from build123d import *

# Parameters (mm, degrees)
SKETCH1_W           = 100
SKETCH1_H           = 40
BOSS_EXTRUDE2_DEPTH = 5
SKETCH4_R           = 3
CUT_EXTRUDE6_DEPTH  = 10
FLEX3_START         = 1.366197724
FLEX3_OUTLINE_W     = 5
FLEX3_OUTLINE_H     = 40
FLEX3_DEPTH         = 48.633802276
FLEX3_START_2       = -3.633802276
FLEX3_2_OUTLINE_W   = 46.366197724
FLEX3_2_OUTLINE_H   = 40
FLEX3_2_OUTLINE_R   = 3
FLEX3_2_DEPTH       = 3.907802276
FLEX3_START_3       = -5
FLEX3_3_OUTLINE_W   = 46.366197724
FLEX3_3_OUTLINE_H   = 40
FLEX3_3_OUTLINE_R   = 3
FLEX3_3_DEPTH       = 6.366197724
FLEX3_START_4       = -40
FLEX3_4_DEPTH       = 40
BOSS_EXTRUDE3_DEPTH = 1.5
CUT_EXTRUDE7_START  = -43
CUT_EXTRUDE7_DEPTH  = 43
BOSS_EXTRUDE4_DEPTH = 1.5
CUT_EXTRUDE8_DEPTH  = 40


with BuildPart() as part:
    # Sketch1 → Boss-Extrude2 (new body)
    with BuildSketch(Plane(origin=(0, 0, 0), x_dir=(1, 0, 0), z_dir=(0, 1, 0))):
        with Locations((0, 20)):
            Rectangle(SKETCH1_W, SKETCH1_H)
    extrude(amount=BOSS_EXTRUDE2_DEPTH)

    # Sketch4 → Cut-Extrude6 (cut)
    with BuildSketch(Plane(origin=(0, 5, 0), x_dir=(1, 0, 0), z_dir=(0, 1, 0))):
        with Locations(Location((-35, 30, 0), (0, 0, 270))):
            Circle(SKETCH4_R)
        with Locations(Location((-35, 10, 0), (0, 0, 270))):
            Circle(SKETCH4_R)
        with Locations(Location((35, 10, 0), (0, 0, 270))):
            Circle(SKETCH4_R)
        with Locations(Location((35, 30, 0), (0, 0, 270))):
            Circle(SKETCH4_R)
    extrude(amount=-CUT_EXTRUDE6_DEPTH, mode=Mode.SUBTRACT)

    # Flex3: read off the stored shape, not the designer's step
    # Flex3 outline → Flex3 (cut)
    with BuildSketch(Plane.YZ.offset(FLEX3_START)):
        with Locations((2.5, -20)):
            Rectangle(FLEX3_OUTLINE_W, FLEX3_OUTLINE_H)
    extrude(amount=FLEX3_DEPTH, mode=Mode.SUBTRACT)

    # Flex3 2 outline → Flex3 2 (add)
    with BuildSketch(Plane.YZ.offset(FLEX3_START_2)):
        with Locations((28.183098862, -20)):
            Rectangle(FLEX3_2_OUTLINE_W, FLEX3_2_OUTLINE_H)
        with Locations((36.366197724, -30)):
            Circle(FLEX3_2_OUTLINE_R, mode=Mode.SUBTRACT)
        with Locations((36.366197724, -10)):
            Circle(FLEX3_2_OUTLINE_R, mode=Mode.SUBTRACT)
    extrude(amount=FLEX3_2_DEPTH)

    # Flex3 3 outline → Flex3 3 (add)
    with BuildSketch(Plane.YZ.offset(FLEX3_START_3)):
        with Locations((28.183098862, -20)):
            Rectangle(FLEX3_3_OUTLINE_W, FLEX3_3_OUTLINE_H)
        with Locations((36.366197724, -30)):
            Circle(FLEX3_3_OUTLINE_R, mode=Mode.SUBTRACT)
        with Locations((36.366197724, -10)):
            Circle(FLEX3_3_OUTLINE_R, mode=Mode.SUBTRACT)
    extrude(amount=FLEX3_3_DEPTH)

    # Flex3 4 outline → Flex3 4 (cut)
    with BuildSketch(Plane.XY.offset(FLEX3_START_4)):
        with BuildLine():
            Line((1.366197724, 0), (1.366197724, 6.366197724))
            ThreePointArc((1.366197724, 6.366197724), (-0.498418419, 1.864616143), (-5, 0))
            Line((-5, 0), (1.366197724, 0))
        make_face()
        with BuildLine():
            ThreePointArc((-5, 5), (-4.033952325, 5.400150049), (-3.633802276, 6.366197724))
            Line((-3.633802276, 6.366197724), (-3.633802276, 51.366197724))
            Line((-3.633802276, 51.366197724), (-5, 51.366197724))
            Line((-5, 51.366197724), (-5, 5))
        make_face()
    extrude(amount=FLEX3_4_DEPTH, mode=Mode.SUBTRACT)

    # Sketch6 → Boss-Extrude3 (add, symmetric)
    with BuildSketch(Plane.XY.offset(-10)):
        Polygon((0, 0), (0, 15), (-15, 0), align=None)
    extrude(amount=BOSS_EXTRUDE3_DEPTH, both=True)

    # Sketch7 → Cut-Extrude7 (cut)
    with BuildSketch(Plane.XY.offset(CUT_EXTRUDE7_START)):
        with BuildLine():
            Line((-5, 0), (0, 0))
            Line((0, 0), (0, 2.425579313))
            ThreePointArc((0, 2.425579313), (-2.221356671, 0.638404544), (-5, 0))
        make_face()
    extrude(amount=CUT_EXTRUDE7_DEPTH, mode=Mode.SUBTRACT)

    # Sketch9 → Boss-Extrude4 (add, symmetric)
    with BuildSketch(Plane.XY.offset(-30)):
        Polygon((0, 0), (0, 15), (-15, 0), align=None)
    extrude(amount=BOSS_EXTRUDE4_DEPTH, both=True)

    # Sketch10 → Cut-Extrude8 (cut)
    with BuildSketch(Plane(origin=(0, 0, -40), x_dir=(-1, 0, 0), z_dir=(0, 0, -1))):
        with BuildLine():
            Line((0, 2.425579313), (0, 0))
            Line((0, 0), (5, 0))
            ThreePointArc((5, 0), (2.221356671, 0.638404544), (0, 2.425579313))
        make_face()
    extrude(amount=-CUT_EXTRUDE8_DEPTH, mode=Mode.SUBTRACT)


solid = part.part
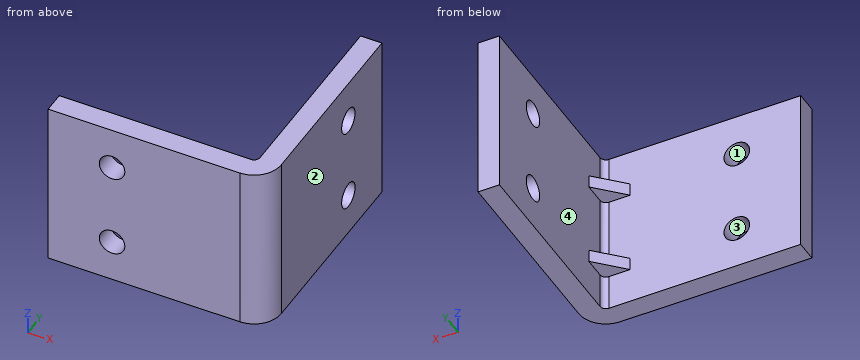
Input: part model. Units: mm. Frame: model coordinates. Face numbers are marked on the shaded views. Coordinates: 2 decimals unless noted, no trailing zeros. Loops run counter-clockwise (first coordinate to the right, second up) from the corner with the lowest first, then second, coordinate; pieces in that order, holes last. Notation, with made-up numbers: (86.5, -10) -> (110.5, -10) arc R20 cw to (110.5, -4) -> close; hole circle Ø4 at (62.25, -26). An arc over 180 degrees is marked (long way). One line per item, written item: value.
(1) Cut plane B-B (x = -35). Output: boundary loops of the cut face in (y, z).
Answer below:
outline: (0, -40) -> (5, -40) -> (5, -33) -> (0, -33) -> close; (0, -27) -> (5, -27) -> (5, -13) -> (0, -13) -> close; (0, -7) -> (5, -7) -> (5, 0) -> (0, 0) -> close
(2) Cut plane D-D (y = 9). Output: boundary loops of the cut face in (x, z), then the cut area to 3 significant figures.
Answer below:
outline: (-6, -31.5) -> (-3.63, -31.5) -> (-3.63, -40) -> (1.37, -40) -> (1.37, 0) -> (-3.63, 0) -> (-3.63, -8.5) -> (-6, -8.5) -> (-6, -11.5) -> (-3.63, -11.5) -> (-3.63, -28.5) -> (-6, -28.5) -> close
area: 214 mm2
(3) Pin query (flat end, axial travel): pin 1 Ø3 at (y, z) = (17.5, -32) entering from -X; pin 2 Ø5 at (x, y) = (-7.5, 9) entering from -Z; pin 3 Ø7 at (x, y) = (-6.5, 7.5) entering from +Z; pin 4 Ø5 at (x, y) = (-8, 9.5) entering from +Z. Return the tip coordinate at first contact, or that it passes through.
Answer below:
pin 1: stops at x = -3.63
pin 2: stops at z = -31.5
pin 3: stops at z = 0
pin 4: stops at z = -8.5
(4) Draft query along X for the marked faces 1, 2, 3 and 4. Return one class per face: pulls with the +X half, pulls with the -X half, needs draft (parallel to the pull), parting line crosses it, or undercut.
Answer below:
face 1: undercut
face 2: pulls with the +X half
face 3: undercut
face 4: pulls with the -X half
(5) Ray query, line 1 along Y through (x, z) = (-20, -16.5); line 2 along X through (y, z) = (10, -23); line 3 along Y through (x, z) = (-2.35, -30). Return the intervals inside material, ascending.
Answer below:
line 1: y = 0 to 5
line 2: x = -3.63 to 1.37
line 3: y = 0.58 to 33.37, 39.37 to 51.37
(6) Cut plane A-A (z = -30). Output: boundary loops of the cut face in (x, y), then the cut area to 3 significant figures.
Answer below:
outline: (-50, 0) -> (-38, 0) -> (-38, 5) -> (-50, 5) -> close; (-32, 0) -> (-5, 0) arc R6.37 ccw to (1.37, 6.37) -> (1.37, 33.37) -> (-3.63, 33.37) -> (-3.63, 11.37) -> (-10, 5) -> (-32, 5) -> close; (-3.63, 39.37) -> (1.37, 39.37) -> (1.37, 51.37) -> (-3.63, 51.37) -> close
area: 440 mm2
(7) Cut plane C-C (y = 35). Output: boundary loops of the cut face in (x, z), then the cut area to 3 significant figures.
Answer below:
outline: (-3.63, -40) -> (1.37, -40) -> (1.37, -32.67) -> (-3.63, -32.67) -> close; (-3.63, -27.33) -> (1.37, -27.33) -> (1.37, -12.67) -> (-3.63, -12.67) -> close; (-3.63, -7.33) -> (1.37, -7.33) -> (1.37, 0) -> (-3.63, 0) -> close
area: 147 mm2
